The listing builds one solid part. Answer for the finished solid, in the listing's coordinates (mm). A direction names the side the tool comes from. Coordinates: 2 decimals unless noted, no trailing zeros. Order: outer loops, then holes, each group sorted by start corner. A loop starts at its lowest first (then second) coordinate and runs counter-clockwise, first axis right, second up. Notation, with made-up numbers: (6, -38) -> (55, -38) arc R20 ccw to (55, -17) -> close; hole circle Ø3 at (52, 20). An arc over 180 degrees is marked (long way). Return JSON: item names as keys, results as strings.
```python
from build123d import *

# Parameters (mm, degrees)
SKETCH_1_R          = 26.37
EXTRUDE_1_DEPTH     = 15
SKETCH_2_R          = 1.65
CUT_EXTRUDE_1_DEPTH = 23


with BuildPart() as part:
    # 草图1 → 凸台-拉伸1 (new body)
    with BuildSketch(Plane(origin=(0, 0, 0), x_dir=(1, 0, 0), z_dir=(0, 1, 0))):
        with BuildLine():
            Line((-40, 7.4), (-29, 7.4))
            Line((-29, 7.4), (-29, -7.4))
            Line((-29, -7.4), (-40, -7.4))
            Line((-40, -7.4), (-40, -10.5))
            Line((-40, -10.5), (-27.182523797, -10.5))
            ThreePointArc((-27.182523797, -10.5), (0, -29.14), (27.182523797, -10.5))
            Line((27.182523797, -10.5), (40, -10.5))
            Line((40, -10.5), (40, -7.4))
            Line((40, -7.4), (29, -7.4))
            Line((29, -7.4), (29, 7.4))
            Line((29, 7.4), (40, 7.4))
            Line((40, 7.4), (40, 10.5))
            Line((40, 10.5), (27.182523797, 10.5))
            ThreePointArc((27.182523797, 10.5), (0, 29.14), (-27.182523797, 10.5))
            Line((-27.182523797, 10.5), (-40, 10.5))
            Line((-40, 10.5), (-40, 7.4))
        make_face()
        Circle(SKETCH_1_R, mode=Mode.SUBTRACT)
    extrude(amount=EXTRUDE_1_DEPTH)

    # 草图2 → 切除-拉伸1 (cut)
    with BuildSketch(Plane(origin=(0, 0, -10.5), x_dir=(-1, 0, 0), z_dir=(0, 0, -1))):
        with Locations((36.5, 7.5)):
            Circle(SKETCH_2_R)
        with Locations((-36.5, 7.5)):
            Circle(SKETCH_2_R)
    extrude(amount=-CUT_EXTRUDE_1_DEPTH, mode=Mode.SUBTRACT)


solid = part.part
```
Item 1: The part is cut by section B-B on x = 0. Determine the outline of the cut face in (y, z).
Answer list:
{"outline": "(0, -29.14) -> (15, -29.14) -> (15, -26.37) -> (0, -26.37) -> close; (0, 26.37) -> (15, 26.37) -> (15, 29.14) -> (0, 29.14) -> close"}
Item 2: Which of the six approach directions +Z, -Z, +X, -X, +Y, -Y give full straight-line access (tool end or side, diameter ignored) to faces 4 (the flat face through (34, 7, -7.4)), 5 (the flat face through (-34, 7, -10.5)), 6 (the flat face through (-34, 7, 10.5))?
Answer list:
{"face 4": "+X, +Y, -Y", "face 5": "-Z, -X, +Y, -Y", "face 6": "+Z, -X, +Y, -Y"}
Item 3: Find the intervals of material crossed by probe 1 along X at (y, z) = (6, 0); probe 2 along Y at (x, z) = (-36.5, 9.5); probe 3 along Z at (x, y) = (-24, 12.5), in increasing order.
Answer list:
{"probe 1": "-29 to -26.37, 26.37 to 29", "probe 2": "0 to 5.85, 9.15 to 15", "probe 3": "-16.53 to -10.93, 10.93 to 16.53"}
Item 4: The part is cut by section A-A on y = 7.5. Count the separate pieces of the cut face and the enclosed holes in it, plus the area to 3 significant figures.
Answer list:
{"separate pieces": "5", "enclosed holes": "1", "area": "600 mm2"}
Item 5: Determine the mould class of faces 1 (the flat face through (-15, 15, -22)), 2 (the flat face through (34, 7, 10.5)), 3 (the cylindrical face through (-34.85, 7.57, -8.97)) for opening direction Y: pulls with the +Y half, pulls with the -Y half, needs draft (parallel to the pull), parting line crosses it, or undercut.
Answer list:
{"face 1": "pulls with the +Y half", "face 2": "needs draft", "face 3": "undercut"}
Item 6: The part is cut by section D-D on z = 0. Determine the outline of the cut face in (x, y).
Answer list:
{"outline": "(-29, 0) -> (-26.37, 0) -> (-26.37, 15) -> (-29, 15) -> close; (26.37, 0) -> (29, 0) -> (29, 15) -> (26.37, 15) -> close"}
Item 7: Flat-ended cylindrical pins translate along their axes: pin 1 (4.5 mm diameter, centred on x = 36.5, y = 7.5, fed in from -Z); pin 2 (3 mm diameter, centred on x = 36.5, y = 7.5, fed in from -Z); pin 3 (1 mm diameter, centred on x = -1.5, y = 12.5, fed in from -Z); pin 4 (3.5 mm diameter, centred on x = 36, y = 6, fed in from +Z). Find the tip coordinate at first contact, or state that the pin passes through.
Answer list:
{"pin 1": "z = -10.5", "pin 2": "through", "pin 3": "z = -29.12", "pin 4": "z = 10.5"}
Item 8: The part is cut by section C-C on x = -36.5. Determine the outline of the cut face in (y, z), plus the area to 3 significant figures.
Answer list:
{"outline": "(0, -10.5) -> (5.85, -10.5) -> (5.85, -7.4) -> (0, -7.4) -> close; (0, 7.4) -> (5.85, 7.4) -> (5.85, 10.5) -> (0, 10.5) -> close; (9.15, -10.5) -> (15, -10.5) -> (15, -7.4) -> (9.15, -7.4) -> close; (9.15, 7.4) -> (15, 7.4) -> (15, 10.5) -> (9.15, 10.5) -> close", "area": "72.5 mm2"}
